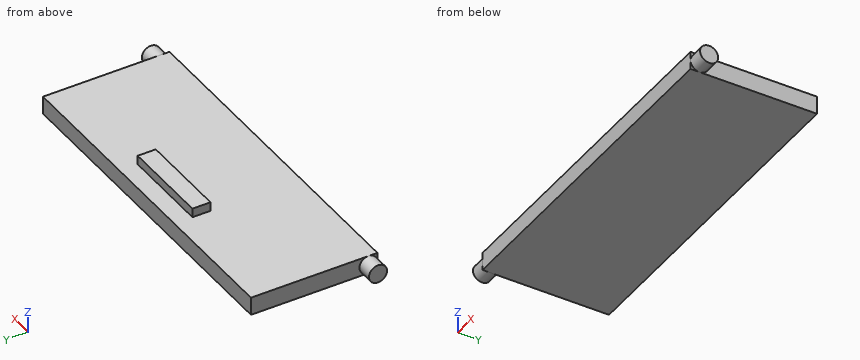
from build123d import *

# Parameters (mm, degrees)
F0_W     = 48.26
F0_H     = 17.78
F1_DEPTH = 2.54
F2_R     = 1.27
F3_DEPTH = 26.3525
F4_W     = 12.7
F4_H     = 2.54
F5_DEPTH = 1.27


with BuildPart() as f1:
    # F0 (on Top) → F1 (new body)
    with BuildSketch(Plane.XY):
        Rectangle(F0_W, F0_H)
    extrude(amount=F1_DEPTH)

    # F2 (on Right) → F3 (join, symmetric)
    with BuildSketch(Plane.YZ):
        with Locations((-7.62, 1.27)):
            Circle(F2_R)
    extrude(amount=F3_DEPTH, both=True)

    # F4 (on face) → F5 (join)
    with BuildSketch(Plane.XY.offset(2.54)):
        with Locations((0, 5.08)):
            Rectangle(F4_W, F4_H)
    extrude(amount=F5_DEPTH)


solid = f1.part
Check sheet for the modelled part. Datum: model origin and axes. Units: mm. Round coordinates to 2 decimals unless told otherwise and drop trailing zeros. Loops run counter-clockwise (first coordinate to the right, second up) from the corner with the lowest first, then second, coordinate; pieces in that order, holes last. Notation, with made-up numbers: M -16.5,84.5 L 34.5,84.5 A34 cw 34.5,122.5 Z; hole C 26,86 d10. An arc over 180 degrees is marked long. One line per question, with ' | ' between items. Start each with the question number.
Item 1: Section check B-B (z = 3). Record the boundary of the cut face in (x, y), and give its area (3 significant figures).
Item 2: Scan lines: probe 1 along X at (y, z) = (3.75, 1); probe 2 along Y at (x, z) = (2, 3.65); probe 3 along Z at (x, y) = (23.5, -8). Record each from-to range of solid material in increasing order.
Item 3: Section check A-A (x = -2). Record the boundary of the cut face in (y, z).
Item 4: Gauge pin test, flat ends, axial feed: pin 1 Ø1 at (y, z) = (4.5, 3) entering from +X; pin 2 Ø1.5 at (y, z) = (6, 2) entering from -X; pin 3 Ø0.6 at (y, z) = (5, 3.5) entering from -X; pin 4 Ø1 at (x, z) = (14.5, 3.5) entering from -Y. Record the tip position at first contact, or that the pin passes through.
Item 5: Section check C-C (y = 2.25). Record the boundary of the cut face in (x, z), and give its area (3 significant figures).
Worked out:
1) outline: M -6.35,3.81 L 6.35,3.81 L 6.35,6.35 L -6.35,6.35 Z | area: 32.3 mm^2
2) probe 1: -24.13 to 24.13 | probe 2: 3.81 to 6.35 | probe 3: 0 to 2.54
3) outline: M -8.89,0 L 8.89,0 L 8.89,2.54 L 6.35,2.54 L 6.35,3.81 L 3.81,3.81 L 3.81,2.54 L -8.89,2.54 Z
4) pin 1: x = 24.13 | pin 2: x = -24.13 | pin 3: x = -6.35 | pin 4: through
5) outline: M -24.13,0 L 24.13,0 L 24.13,2.54 L -24.13,2.54 Z | area: 123 mm^2
